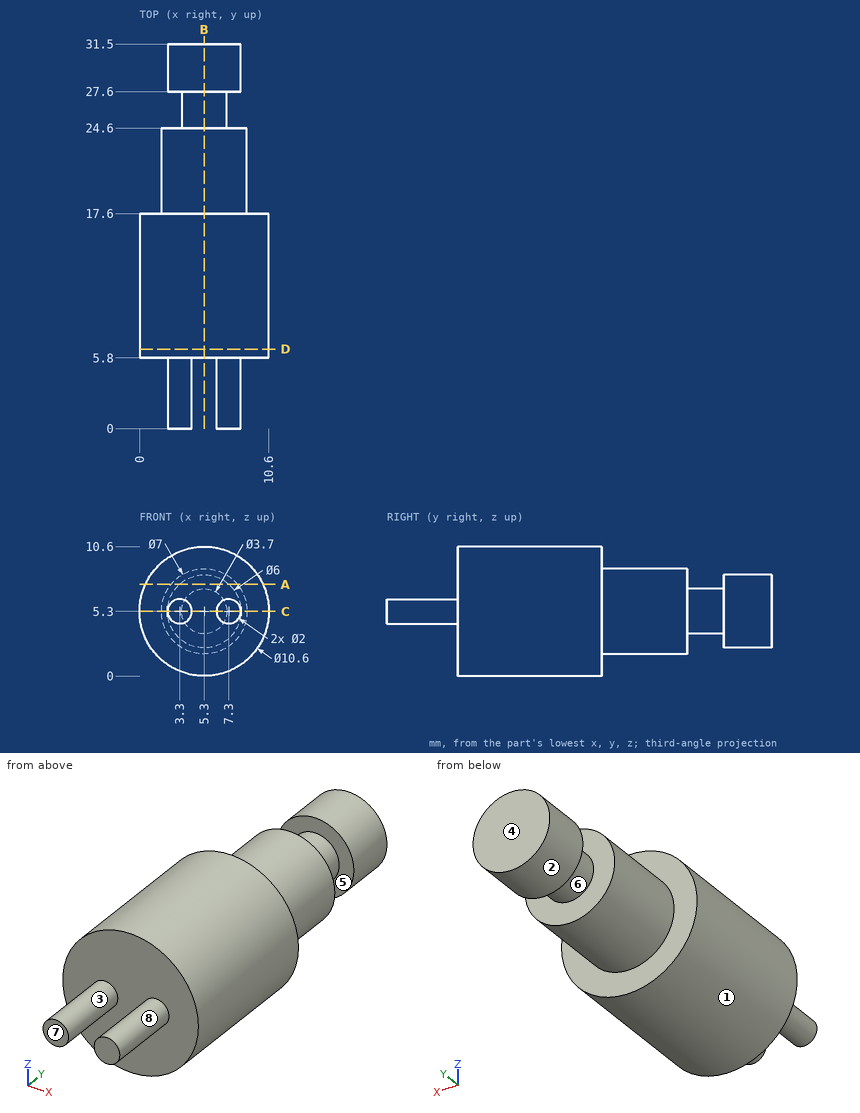
Verification items for this drawing (mm, ordinates from the low corner). A direction names the side the tool comes from. Coordinates: 2 decimals unless noted, no trailing zeros. Write each loop counter-clockwise with the first axis right and the second up, starting at its lowest first coordinate (ties: lowest second). Pieces come first, ordered by that corner, then holes. Notation, with made-up numbers: M 22.5,-13.5 L 52.5,-13.5 A18 ccw 52.5,4.5 Z; hole C 86.5,-35 d2. An arc over 180 degrees is marked long. Answer as a JSON object with one key per item and string values.
1. Section check D-D, the plane y = 6.5. Enter the section's corners in (x, z), plus the area to 3 significant figures.
Answers below:
{"outline": "C 5.3,5.3 d10.6", "area": "88.2 mm²"}
2. Section check C-C, the plane z = 5.3. Enter the section's corners in (x, y).
Answers below:
{"outline": "M 0,5.8 L 2.3,5.8 L 2.3,0 L 4.3,0 L 4.3,5.8 L 6.3,5.8 L 6.3,0 L 8.3,0 L 8.3,5.8 L 10.6,5.8 L 10.6,17.6 L 8.8,17.6 L 8.8,24.6 L 7.15,24.6 L 7.15,27.6 L 8.3,27.6 L 8.3,31.5 L 2.3,31.5 L 2.3,27.6 L 3.45,27.6 L 3.45,24.6 L 1.8,24.6 L 1.8,17.6 L 0,17.6 Z"}
3. Draft check along X on the marked faces 6, 7 and 8. Enter one of: released by +X, released by -X, zero draft, split by the parting line, or undercut.
Answers below:
{"face 6": "split by the parting line", "face 7": "zero draft", "face 8": "undercut"}
4. Section check A-A, the plane z = 7.5. Enter the section's corners in (x, y).
Answers below:
{"outline": "M 0.48,5.8 L 10.12,5.8 L 10.12,17.6 L 8.02,17.6 L 8.02,24.6 L 2.58,24.6 L 2.58,17.6 L 0.48,17.6 Z; M 3.26,27.6 L 7.34,27.6 L 7.34,31.5 L 3.26,31.5 Z"}
5. Go/stop test with flat-tipped pins: pin 1 Ø5 at (x, y) = (8.5, 4) entering from +Z; pin 2 Ø2 at (x, y) = (7.5, 24) entering from +Z; pin 3 Ø3 at (x, y) = (2, 4) entering from +Z. Record where each tip stops, or that it passes through.
Answers below:
{"pin 1": "stops at z = 10.39", "pin 2": "stops at z = 8.59", "pin 3": "stops at z = 6.3"}
6. Scan lines: L1, parallel to Y at x = 5.75, z = 7.75; L2, parallel to Y at x = 3, z = 1.5; L3, parallel to Y at x = 5.5, z = 6. Record each from-to range of solid material in increasing order.
Answers below:
{"L1": "y = 5.8 to 24.6, 27.6 to 31.5", "L2": "y = 5.8 to 17.6", "L3": "y = 5.8 to 31.5"}
7. Tool access check on the marked faces 1, 2, 3, 4 and 5. Record the directions out of +Z, -Z, +X, -X, +Y, -Y that give a thin tool (end or side, any length) a straight path to the whole face; none if there is none.
Answers below:
{"face 1": "+Y, -Y", "face 2": "+Y", "face 3": "-Y", "face 4": "+Z, -Z, +X, -X, +Y", "face 5": "none"}
8. Section check B-B, the plane x = 5.3. Enter the section's corners in (y, z).
Answers below:
{"outline": "M 5.8,0 L 17.6,0 L 17.6,1.8 L 24.6,1.8 L 24.6,3.45 L 27.6,3.45 L 27.6,2.3 L 31.5,2.3 L 31.5,8.3 L 27.6,8.3 L 27.6,7.15 L 24.6,7.15 L 24.6,8.8 L 17.6,8.8 L 17.6,10.6 L 5.8,10.6 Z"}
